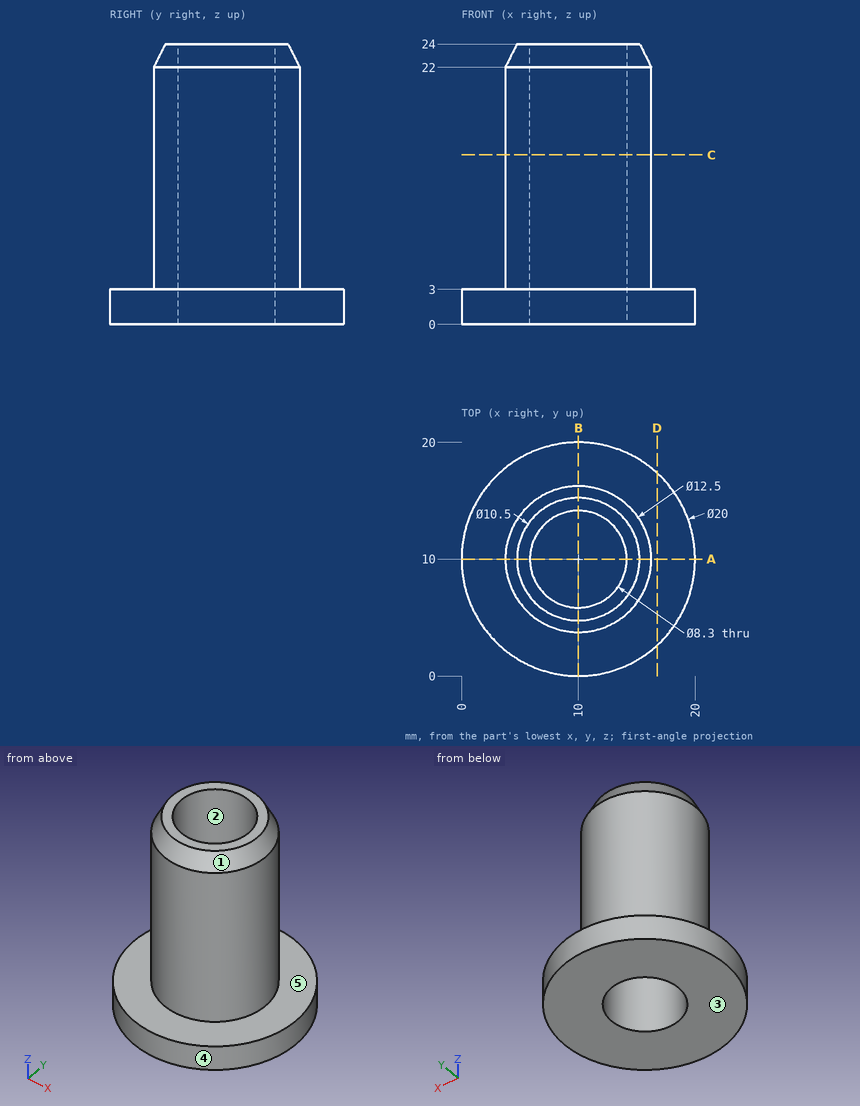
Geometry: see drawing. Coordinates: mm, zero at the bounding-box minimum. A direction names the side the tool comes from. Coordinates: 2 decimals unless noted, no trailing zeros. Loops run counter-clockwise (first coordinate to the right, second up) from the corner with the lowest first, then second, coordinate; pieces in that order, holes last. Notation, with made-up numbers: M 43,-13.75 L 61,-13.75 A20 ccw 61,18.25 Z; hole C 57,-29.5 d8. An arc over 180 degrees is marked long. Answer in a Markdown table with one row per item.
1. Reachability of the marked faces 4 and 5 from +Z, -Z, +X, -X, +Y, -Y: full face, straight path, thin tool, end or side. Return the list, or none.
Response:
| item | result |
|---|---|
| face 4 | +Z, -Z |
| face 5 | +Z |
2. Section C-C, the plane z = 14.5. Output: boundary loops of the cut face in (x, y), then the cut area to 3 significant figures.
Response:
| item | result |
|---|---|
| outline | C 10,10 d12.5; hole C 10,10 d8.3 |
| area | 68.6 mm2 |
3. Section D-D, the plane x = 16.75. Output: boundary loops of the cut face in (y, z).
Response:
| item | result |
|---|---|
| outline | M 2.62,0 L 17.38,0 L 17.38,3 L 2.62,3 Z |
4. Material intervals for line 1 (Y direction, x = 10, z = 8); line 2 (Z direction, x = 19.25, y = 11.75); line 3 (Y direction, x = 8, z = 18.5), sorted ascending.
Response:
| item | result |
|---|---|
| line 1 | y = 3.75 to 5.85, 14.15 to 16.25 |
| line 2 | z = 0 to 3 |
| line 3 | y = 4.08 to 6.36, 13.64 to 15.92 |
5. Draft query along X for the marked faces 1, 2 and 3. Return one class per face: pulls with the +X half, pulls with the -X half, needs draft (parallel to the pull), parting line crosses it, or undercut.
Response:
| item | result |
|---|---|
| face 1 | parting line crosses it |
| face 2 | undercut |
| face 3 | needs draft |
6. First-contact query: pin 1 (1.5 mm diameter, centred on x = 3.5, z = 13, fed in from -Y); pin 2 (6 mm diameter, centred on x = 16, y = 3, fed in from +Z); pin 3 (3 mm diameter, centred on x = 15, z = 11.5, fed in from +Y). Flat tips, straight axial feed; report the tip coordinate or a pass-through.
Response:
| item | result |
|---|---|
| pin 1 | stops at y = 7.55 |
| pin 2 | stops at z = 22.06 |
| pin 3 | stops at y = 15.18 |
7. Section A-A, the plane y = 10. Output: boundary loops of the cut face in (x, z).
Response:
| item | result |
|---|---|
| outline | M 0,0 L 5.85,0 L 5.85,24 L 4.75,24 L 3.75,22 L 3.75,3 L 0,3 Z; M 14.15,0 L 20,0 L 20,3 L 16.25,3 L 16.25,22 L 15.25,24 L 14.15,24 Z |
